from build123d import *

# Parameters (mm, degrees)
SKETCH1_R           = 17.5
SKETCH1_R_2         = 4
SKETCH1_R_3         = 1.5
BOSS_EXTRUDE1_DEPTH = 4
BOSS_EXTRUDE2_DEPTH = 10
SKETCH3_R           = 4
CUT_EXTRUDE1_DEPTH  = 10


with BuildPart() as part:
    # Sketch1 → Boss-Extrude1 (new body)
    with BuildSketch(Plane(origin=(0, 0, 0), x_dir=(1, 0, 0), z_dir=(0, 1, 0))):
        with Locations(Location((0, 0, 0), (0, 0, 270))):
            Circle(SKETCH1_R)
        with Locations(Location((0, 0, 0), (0, 0, 270))):
            Circle(SKETCH1_R_2, mode=Mode.SUBTRACT)
        with Locations(Location((-12.5, 0, 0), (0, 0, 270))):
            Circle(SKETCH1_R_3, mode=Mode.SUBTRACT)
        with Locations(Location((0, 12.5, 0), (0, 0, 270))):
            Circle(SKETCH1_R_3, mode=Mode.SUBTRACT)
        with Locations(Location((12.5, 0, 0), (0, 0, 270))):
            Circle(SKETCH1_R_3, mode=Mode.SUBTRACT)
        with Locations(Location((0, -12.5, 0), (0, 0, 270))):
            Circle(SKETCH1_R_3, mode=Mode.SUBTRACT)
    extrude(amount=BOSS_EXTRUDE1_DEPTH)

    # Sketch2 → Boss-Extrude2 (add)
    with BuildSketch(Plane(origin=(0, 4, 0), x_dir=(1, 0, 0), z_dir=(0, 1, 0))):
        with BuildLine():
            Line((-6.25, -6.25), (-9.785533906, -2.714466094))
            Line((-9.785533906, -2.714466094), (-15.394075132, -8.32300732))
            ThreePointArc((-15.394075132, -8.32300732), (-12.374368671, -12.374368671), (-8.32300732, -15.394075132))
            Line((-8.32300732, -15.394075132), (-2.714466094, -9.785533906))
            Line((-2.714466094, -9.785533906), (-6.25, -6.25))
        make_face()
    extrude(amount=BOSS_EXTRUDE2_DEPTH)

    # Sketch3 → Cut-Extrude1 (cut)
    with BuildSketch(Plane(origin=(-6.25, 0, 6.25), x_dir=(-0.7071067811865475, 0, -0.7071067811865477), z_dir=(0.7071067811865477, 0, -0.7071067811865475))):
        with Locations((0, 14)):
            Circle(SKETCH3_R)
    extrude(amount=-CUT_EXTRUDE1_DEPTH, mode=Mode.SUBTRACT)


solid = part.part
CAD build for the part. Positions are in the model's coordinates, mm. A direction names the side the tool comes from. Give positions to 0.01 mm unless a question says otherwise; leave off trailing zeros. Order: outer loops, then holes, each group sorted by start corner. A loop starts at its lowest first (then second) coordinate and runs counter-clockwise, first axis right, second up. Notation, with made-up numbers: (38.25, 42) - (42.25, 42) arc R9 cw to (42.25, 54) - close; hole circle Ø9 at (50, 42). An arc over 180 degrees is marked (long way). Answer in a Markdown table with one row per item.
1. Saw through at D-D, the plane y = 12.5. Give the cut face in (x, z), plus the area to 3 significant figures.
Data:
| item | result |
|---|---|
| outline | (-15.39, 8.32) - (-9.79, 2.71) - (-8.87, 3.63) - (-14.72, 9.47) arc R17.5 ccw to start; (-9.47, 14.72) - (-3.63, 8.87) - (-2.71, 9.79) - (-8.32, 15.39) arc R17.5 ccw to start |
| area | 20.9 mm² |
2. Saw through at A-A, the plane z = 0. Give the cut face in (x, y), plus the area to 3 significant figures.
Data:
| item | result |
|---|---|
| outline | (-17.5, 0) - (-14, 0) - (-14, 4) - (-17.5, 4) - close; (-11, 0) - (-4, 0) - (-4, 4) - (-11, 4) - close; (4, 0) - (11, 0) - (11, 4) - (4, 4) - close; (14, 0) - (17.5, 0) - (17.5, 4) - (14, 4) - close |
| area | 84.0 mm² |
3. Probe probe 1 along X at (y, z) = (1.95, 0); probe 2 along Y at (x, z) = (5, -4); probe 3 along Z at (x, y) = (-10.5, 7). List the from-to ranges inside material, lowest first. Write a range as [from, to].
Data:
| item | result |
|---|---|
| probe 1 | x = [-17.5, -14], [-11, -4], [4, 11], [14, 17.5] |
| probe 2 | y = [0, 4] |
| probe 3 | z = [3.43, 14] |
4. Tool access for faces 4 (the flat face through (-6.2, 7.8, 6.3)), 5 (the cylindrical face through (-12.05, 1.97, 1.43)): list every direction of +Z, -Z, +X, -X, +Y, -Y with a clear straight run to the whole face (end or side of a thin tool).
Data:
| item | result |
|---|---|
| face 4 | -Z, +X, +Y |
| face 5 | +Y, -Y |
5. Saw through at C-C, the plane y = 3.25. Give the cut face in (x, z), plus the area to 3 significant figures.
Data:
| item | result |
|---|---|
| outline | circle Ø35 at (0, 0); hole circle Ø3 at (-12.5, 0); hole circle Ø8 at (0, 0); hole circle Ø3 at (0, -12.5); hole circle Ø3 at (0, 12.5); hole circle Ø3 at (12.5, 0) |
| area | 884 mm² |
6. Saw through at B-B, the plane x = 0. Give the cut face in (y, z), plus the area to 3 significant figures.
Data:
| item | result |
|---|---|
| outline | (0, -17.5) - (4, -17.5) - (4, -14) - (0, -14) - close; (0, -11) - (4, -11) - (4, -4) - (0, -4) - close; (0, 4) - (4, 4) - (4, 11) - (0, 11) - close; (0, 14) - (4, 14) - (4, 17.5) - (0, 17.5) - close |
| area | 84.0 mm² |
7. Flat gauge pins, fed straight in: pin 1 (10.5 mm diameter, centred on x = 8.5, z = 1.5, fed in from +Y); pin 2 (6 mm diameter, centred on y = 6.5, z = -10, fed in from +X). Where does each tip first touch, or does it go through?
Data:
| item | result |
|---|---|
| pin 1 | stops at y = 4 |
| pin 2 | stops at x = 15.38 |
8. Pull direction X, two halves, no side cores. Call faces 1 (the cylindrical face through (0, 2, -14)), 2 (the flat face through (-12.55, 8.93, 5.48)), 3 (the flat face through (-5.56, 8.93, 12.63)): pulls with the +X half, pulls with the -X half, needs draft (parallel to the pull), parting line crosses it, or undercut.
Data:
| item | result |
|---|---|
| face 1 | undercut |
| face 2 | pulls with the -X half |
| face 3 | pulls with the +X half |
